Work out the finished part from the listing and answer in its coordinate system (mm). A direction names the side the tool comes from. Round coordinates to 2 decimals unless told otherwise and drop trailing zeros. Write each loop counter-clockwise with the first axis right and the second up, starting at its lowest first coordinate (ties: lowest second). Pieces come first, ordered by that corner, then holes. Notation, with made-up numbers: M -12.5,6 L 40.5,6 A21 ccw 40.5,14 Z; hole C 23.25,67.25 d10. An arc over 180 degrees is marked long. Answer in a Markdown table with one row per item.
```python
from build123d import *

# Parameters (mm, degrees)
SKETCH_W        = 75
SKETCH_H        = 18
PAD_DEPTH       = 5
SKETCH001_W     = 50
SKETCH001_H     = 4
POCKET_DEPTH    = 5.001
SKETCH002_W     = 75
SKETCH002_H     = 5
PAD001_DEPTH    = 38
POCKET001_DEPTH = 5
SKETCH004_R     = 11
POCKET002_DEPTH = 5.001
SKETCH005_R     = 10.5
PAD002_DEPTH    = 6
SKETCH006_W     = 10
SKETCH006_H     = 18
PAD003_DEPTH    = 14
SKETCH007_R     = 3
POCKET003_DEPTH = 15
SKETCH008_R     = 16
SKETCH008_R_2   = 7
PAD004_DEPTH    = 1
SKETCH009_R     = 1.75
POCKET004_DEPTH = 18.001
SKETCH010_R     = 4
POCKET005_DEPTH = 8
SKETCH011_R     = 1.75
POCKET006_DEPTH = 18.001
SKETCH012_W     = 100
SKETCH012_H     = 30
POCKET007_DEPTH = 6
SKETCH013_R     = 1.25
HOLE_DEPTH      = 25


with BuildPart() as part:
    # Sketch → Pad (new body)
    with BuildSketch(Plane.XY):
        with Locations((37.5, 9)):
            Rectangle(SKETCH_W, SKETCH_H)
    extrude(amount=PAD_DEPTH)

    # Sketch001 (on Face6 of Pad) → Pocket (cut, through all)
    with BuildSketch(Plane.XY.offset(5)):
        with Locations((37.5, 9)):
            Rectangle(SKETCH001_W, SKETCH001_H)
    extrude(amount=-POCKET_DEPTH, mode=Mode.SUBTRACT)

    # Sketch002 (on Face5 of Pocket) → Pad001 (join)
    with BuildSketch(Plane.XY.offset(5)):
        with Locations((37.5, 15.5)):
            Rectangle(SKETCH002_W, SKETCH002_H)
    extrude(amount=PAD001_DEPTH)

    # Sketch003 (on Face13 of Pad001) → Pocket001 (cut)
    with BuildSketch(Plane.XZ.offset(-13)):
        with BuildLine():
            ThreePointArc((56.5, 19), (37.5, 38), (18.5, 19))
            Line((18.5, 19), (-1.5, 19))
            Line((-1.5, 19), (-1.5, 49))
            Line((-1.5, 49), (76.5, 49))
            Line((76.5, 49), (76.5, 19))
            Line((76.5, 19), (56.5, 19))
        make_face()
    extrude(amount=-POCKET001_DEPTH, mode=Mode.SUBTRACT)

    # Sketch004 → Pocket002 (cut, through all)
    with BuildSketch(Plane.XZ.offset(-13)):
        with Locations((37.5, 19)):
            Circle(SKETCH004_R)
    extrude(amount=-POCKET002_DEPTH, mode=Mode.SUBTRACT)

    # Sketch005 (on Face1 of Pocket002) → Pad002 (join)
    with BuildSketch(Plane.XZ):
        with BuildLine():
            Line((56.5, 19), (75, 19))
            Line((75, 19), (75, 0))
            Line((75, 0), (0, 0))
            Line((0, 0), (0, 19))
            Line((0, 19), (18.5, 19))
            ThreePointArc((56.5, 19), (37.5, 38), (18.5, 19))
        make_face()
        with Locations((37.5, 19)):
            Circle(SKETCH005_R, mode=Mode.SUBTRACT)
    extrude(amount=-PAD002_DEPTH)

    # Sketch006 (on Face8 of Pad002) → Pad003 (join)
    with BuildSketch(Plane.XY.offset(5)):
        with Locations((5, 9)):
            Rectangle(SKETCH006_W, SKETCH006_H)
        with Locations((70, 9)):
            Rectangle(SKETCH006_W, SKETCH006_H)
    extrude(amount=PAD003_DEPTH)

    # Sketch007 (on Face23 of Pad003) → Pocket003 (cut)
    with BuildSketch(Plane.XY.offset(19)):
        with Locations((5, 9.260643)):
            Circle(SKETCH007_R)
        with Locations((70, 9.622806)):
            Circle(SKETCH007_R)
    extrude(amount=-POCKET003_DEPTH, mode=Mode.SUBTRACT)

    # Sketch008 (on Face35 of Pad003) → Pad004 (join)
    with BuildSketch(Plane(origin=(0, 6, 0), x_dir=(-1, 0, 0), z_dir=(0, 1, 0))):
        with Locations((-37.5, 19)):
            Circle(SKETCH008_R)
        with Locations((-37.5, 19)):
            Circle(SKETCH008_R_2, mode=Mode.SUBTRACT)
    extrude(amount=-PAD004_DEPTH)

    # Sketch009 (on Face31 of Pad004) → Pocket004 (cut, through all)
    with BuildSketch(Plane.XZ):
        with Locations((5, 12)):
            Circle(SKETCH009_R)
        with Locations((70, 12)):
            Circle(SKETCH009_R)
    extrude(amount=-POCKET004_DEPTH, mode=Mode.SUBTRACT)

    # Sketch010 (on Face34 of Pocket004) → Pocket005 (cut)
    with BuildSketch(Plane.XZ):
        with Locations((37.5, 5)):
            Circle(SKETCH010_R)
        with Locations((25.375644, 26)):
            Circle(SKETCH010_R)
        with Locations((49.624356, 26)):
            Circle(SKETCH010_R)
    extrude(amount=-POCKET005_DEPTH, mode=Mode.SUBTRACT)

    # Sketch011 (on Face34 of Pocket005) → Pocket006 (cut, through all)
    with BuildSketch(Plane.XZ):
        with Locations((25.375644, 26)):
            Circle(SKETCH011_R)
        with Locations((37.5, 5)):
            Circle(SKETCH011_R)
        with Locations((49.624356, 26)):
            Circle(SKETCH011_R)
    extrude(amount=-POCKET006_DEPTH, mode=Mode.SUBTRACT)

    # Sketch012 (on Face40 of Pocket006) → Pocket007 (cut)
    with BuildSketch(Plane.XZ):
        with Locations((50, 34)):
            Rectangle(SKETCH012_W, SKETCH012_H)
    extrude(amount=-POCKET007_DEPTH, mode=Mode.SUBTRACT)

    # Sketch013 (on Face60 of Pocket007) → Hole (cut)
    with BuildSketch(Plane.XY.offset(19)):
        with Locations((14.5, 3)):
            Circle(SKETCH013_R)
        with Locations((60.5, 3)):
            Circle(SKETCH013_R)
    extrude(amount=-HOLE_DEPTH, mode=Mode.SUBTRACT)


solid = part.part
```
1. The part is cut by section D-D (x = 37.5). Determine the outline of the cut face in (y, z), plus the area to 3 significant figures.
Calculated:
| item | result |
|---|---|
| outline | M 0,0 L 7,0 L 7,1 L 0,1 Z; M 5,9 L 6,9 L 6,12 L 5,12 Z; M 11,0 L 18,0 L 18,3.25 L 11,3.25 Z; M 13,6.75 L 18,6.75 L 18,8 L 13,8 Z; M 13,30 L 18,30 L 18,38 L 13,38 Z |
| area | 79.0 mm² |
2. Determine the mould class of faces 4 (the cylindrical face through (61.69, 3.38, 9.63)), 5 (the cylindrical face through (37.918, 15.465, 37.995)), 6 (the flat face through (8.3, 8.9, 19)) for opening direction X: released by +X, released by -X, zero draft, split by the parting line, or undercut.
Calculated:
| item | result |
|---|---|
| face 4 | undercut |
| face 5 | split by the parting line |
| face 6 | zero draft |
3. The part is cut by section B-B (y = 16.25). Determine the outline of the cut face in (x, z).
Calculated:
| item | result |
|---|---|
| outline | M 0,0 L 75,0 L 75,19 L 56.5,19 A19 ccw 18.5,19 L 0,19 Z; hole C 5,12 d3.5; hole C 25.38,26 d3.5; hole C 37.5,19 d22; hole C 37.5,5 d3.5; hole C 49.62,26 d3.5; hole C 70,12 d3.5 |
4. The part is cut by section A-A (x = 5). Determine the outline of the cut face in (y, z).
Calculated:
| item | result |
|---|---|
| outline | M 0,0 L 18,0 L 18,10.25 L 12.26,10.25 L 12.26,4 L 6.26,4 L 6.26,10.25 L 0,10.25 Z; M 0,13.75 L 6.26,13.75 L 6.26,19 L 0,19 Z; M 12.26,13.75 L 18,13.75 L 18,19 L 12.26,19 Z |
5. A tool of negligible diameter and unlimited length cuts with its end or side. For faces 1 (the flat face through (20, 12, 5)), 2 (the cylindrical face through (29.44, 2.46, 12.27)), 3 (the flat face through (62.5, 9, 3)), from which of +Z, -Z, +X, -X, +Y, -Y can it reach the whole face along a straight path? Write none if from no direction.
Calculated:
| item | result |
|---|---|
| face 1 | +Z |
| face 2 | +Z, -Y |
| face 3 | +Z, -Z |
6. Given pin 1 (6.5 mm diameter, centred on x = 37.5, z = 5, fed in from -Y); pin 2 (9 mm diameter, centred on x = 61.5, y = 9.5, fed in from +Z); pin 3 (4 mm diameter, centred on y = 13.5, z = 28.5, fed in from +X); pin 4 (5.5 mm diameter, centred on x = 5, z = 12, fed in from -Y), each flat-ended and moving along its own axis, determine where each tip first touches the part or whether it passes through.
Calculated:
| item | result |
|---|---|
| pin 1 | stops at y = 11 |
| pin 2 | stops at z = 19 |
| pin 3 | stops at x = 54.96 |
| pin 4 | stops at y = 0 |
7. The part is cut by section C-C (z = 16.5). Determine the outline of the cut face in (x, y).
Calculated:
| item | result |
|---|---|
| outline | M 0,0 L 27.3,0 L 27.3,5 L 30.96,5 L 30.96,6 L 10,6 L 10,13 L 26.79,13 L 26.79,18 L 0,18 Z; M 44.04,5 L 47.7,5 L 47.7,0 L 75,0 L 75,18 L 48.21,18 L 48.21,13 L 65,13 L 65,6 L 44.04,6 Z; hole C 5,9.26 d6; hole C 14.5,3 d2.5; hole C 60.5,3 d2.5; hole C 70,9.62 d6 |
8. Consider line 1 along Z through (x, y) = (37.5, 14.5); line 2 along Z through (x, y) = (5, 15.75); line 3 along Y through (x, z) = (64, 10). Determine where each line is inside the solid, lowest interval first. Write a range as from..to.
Calculated:
| item | result |
|---|---|
| line 1 | z = 0..3.25, 6.75..8, 30..38 |
| line 2 | z = 0..10.25, 13.75..19 |
| line 3 | y = 0..6, 13..18 |
